Verification items for this drawing (mm, ordinates from the low corner). Coordinates: 2 decimals unless noted, no trailing zeros. Write each loop counter-clockwise with the first axis right and the second up, starting at its lowest first coordinate (ties: lowest second). Pieces come first, ordered by that corner, then holes. Notation, with made-up numbers: M 59.5,-9 L 73.5,-9 A21 ccw 73.5,15 Z; hole C -38.75,29 d3. An arc over 180 degrees is marked long. Answer as CSV lines item,"result". Start each with the question number.
1) Go/stop test with flat-tipped pins: pin 1 Ø8 at (x, z) = (10, 10) entering from +Y; pin 2 Ø1 at (x, y) = (13, 1.5) entering from -Z; pin 3 Ø1.5 at (x, y) = (11.5, 3) entering from +Z. Record where each tip stops, or that it passes through.
2) Draft check along X on the marked faces 1, 2 and 3. Enter one of: +X half, -X half, draft (parallel to the pull), parting line (faces both ways), or undercut.
3) Section check D-D (y = 2.65). Record the cut outline in (x, z), and give its area (3 significant figures).
4) Section check C-C (x = 17.25). Record the cut outline in (y, z), and give its area (3 significant figures).
5) Material ranges on L1, parallel to Z at x = 10, y = 1.95; L2, parallel to Y at x = 1, z = 12.25; L3, parallel to X at y = 2.35, z = 11.5, recorded low to high. Write a range as [from, to].
6) Section check B-B (x = 10). Record the cut outline in (y, z), and give its area (3 significant figures).
7) Section check A-A (z = 10). Record the cut outline in (x, y).
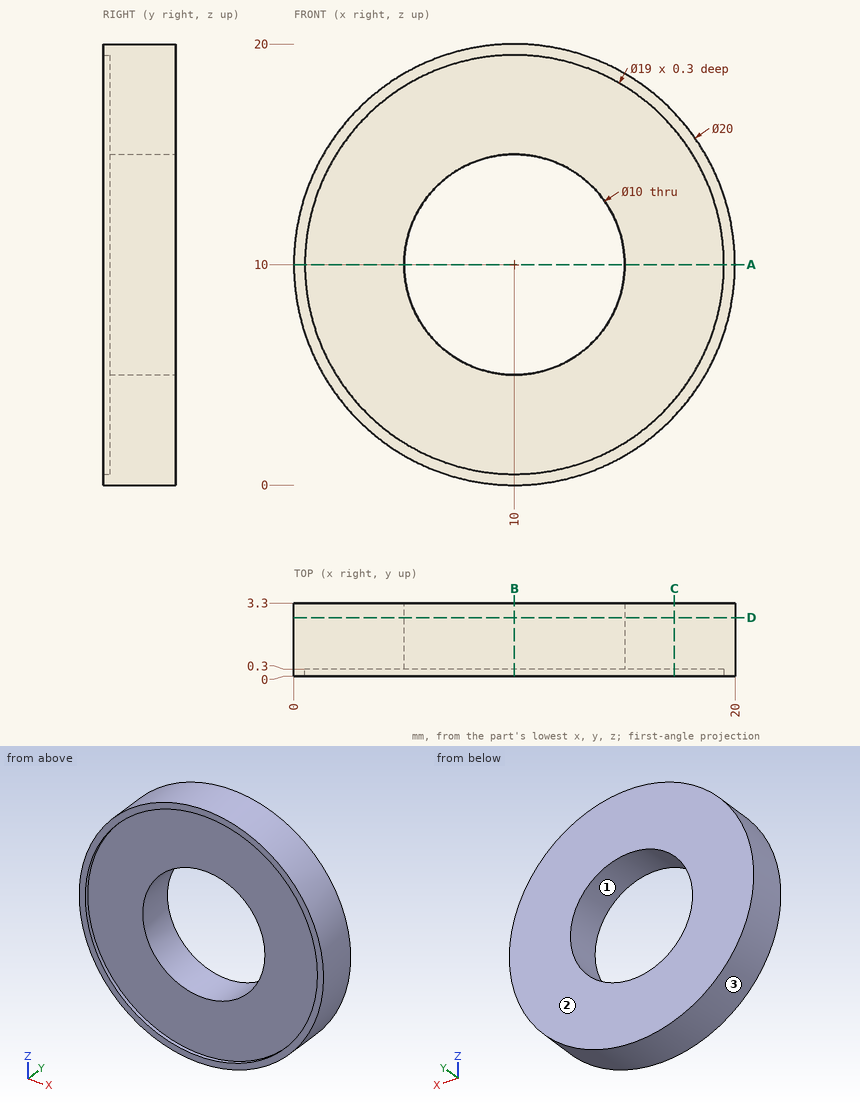
Results found:
1,pin 1,"passes through"
1,pin 2,"stops at z = 0.32"
1,pin 3,"stops at z = 19.97"
2,face 1,"undercut"
2,face 2,"draft"
2,face 3,"parting line"
3,outline,"C 10,10 d20; hole C 10,10 d10"
3,area,"236 mm2"
4,outline,"M 0,3.11 L 3.3,3.11 L 3.3,16.89 L 0,16.89 L 0,16.14 L 0.3,16.14 L 0.3,3.86 L 0,3.86 Z"
4,area,"41.8 mm2"
5,L1,"z = [0, 5], [15, 20]"
5,L2,"y = [0.3, 3.3]"
5,L3,"x = [0.11, 5.23], [14.77, 19.89]"
6,outline,"M 0,0 L 3.3,0 L 3.3,5 L 0.3,5 L 0.3,0.5 L 0,0.5 Z; M 0,19.5 L 0.3,19.5 L 0.3,15 L 3.3,15 L 3.3,20 L 0,20 Z"
6,area,"30.3 mm2"
7,outline,"M 0,0 L 0.5,0 L 0.5,0.3 L 5,0.3 L 5,3.3 L 0,3.3 Z; M 15,0.3 L 19.5,0.3 L 19.5,0 L 20,0 L 20,3.3 L 15,3.3 Z"
